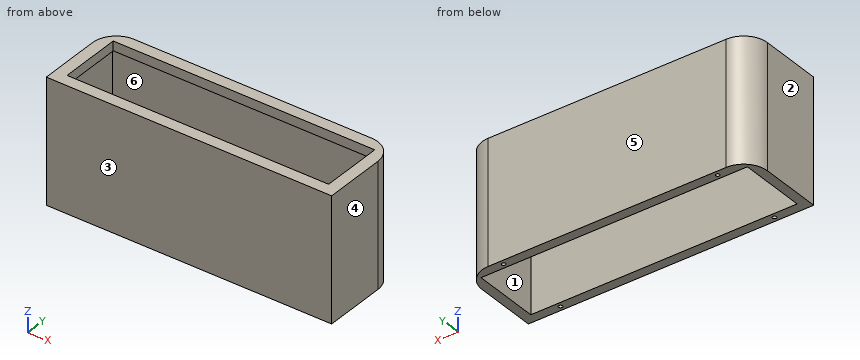
```python
from build123d import *

# Parameters (mm, degrees)
SKETCH1_W           = 152.4
SKETCH1_H           = 45.72
BOSS_EXTRUDE2_DEPTH = 66.04
SHELL1_T            = -5.08
SKETCH2_W           = 139.7
SKETCH2_H           = 33.02
CUT_EXTRUDE1_DEPTH  = 13.462
FILLET1_R           = 12.7
SKETCH4_R           = 1
CUT_EXTRUDE2_DEPTH  = 3.175


with BuildPart() as part:
    # Sketch1 → Boss-Extrude2 (new body)
    with BuildSketch(Plane.XY):
        Rectangle(SKETCH1_W, SKETCH1_H)
    extrude(amount=BOSS_EXTRUDE2_DEPTH)

    # Shell1
    shell1_openings = [part.faces().sort_by_distance(p)[0] for p in [
        (0, 0, 0),
    ]]
    offset(amount=SHELL1_T, openings=shell1_openings, kind=Kind.INTERSECTION)

    # Sketch2 → Cut-Extrude1 (cut)
    with BuildSketch(Plane.XY.offset(66.04)):
        Rectangle(SKETCH2_W, SKETCH2_H)
    extrude(amount=-CUT_EXTRUDE1_DEPTH, mode=Mode.SUBTRACT)

    # Fillet1
    fillet1_edges = [part.edges().sort_by_distance(p)[0] for p in [
        (-76.2, 22.86, 33.02),
        (76.2, 22.86, 33.02),
    ]]
    fillet(fillet1_edges, radius=FILLET1_R)

    # Sketch4 → Cut-Extrude2 (cut)
    with BuildSketch(Plane(origin=(0, 0, 0), x_dir=(-1, 0, 0), z_dir=(0, 0, -1))):
        with Locations((-57.15, -20.32)):
            Circle(SKETCH4_R)
        with Locations((-57.15, 20.32)):
            Circle(SKETCH4_R)
        with Locations((57.15, 20.32)):
            Circle(SKETCH4_R)
        with Locations((57.15, -20.32)):
            Circle(SKETCH4_R)
    extrude(amount=-CUT_EXTRUDE2_DEPTH, mode=Mode.SUBTRACT)


solid = part.part
```
Design review of the part built by this model. Coordinates are the model's own, in mm. Face numbers are marked on the shaded views. A direction names the side the tool comes from. Coordinates: 2 decimals unless noted, no trailing zeros. Loops run counter-clockwise (first coordinate to the right, second up) from the corner with the lowest first, then second, coordinate; pieces in that order, holes last. Notation, with made-up numbers: (66, 82.25) -> (85, 82.25) arc R17 cw to (85, 94.25) -> close; hole circle Ø8 at (10.5, 24.5). An arc over 180 degrees is marked (long way). Answer as a JSON object with one key per item and string values.
Q1. To check wall thickness, follow L1, parallel to Y at x = 57, z = 1; L2, parallel to X at y = -8, z = 39; L3, parallel to X at y = 20, z = 1. State the ranges of each line that lie inside material, in increasing order.
Answer block:
{"L1": "y = -22.86 to -21.31, -19.33 to -17.78, 17.78 to 19.33, 21.31 to 22.86", "L2": "x = -76.2 to -71.12, 71.12 to 76.2", "L3": "x = -71.53 to -58.1, -56.2 to 56.2, 58.1 to 71.53"}
Q2. The part is to be moulded in two halves that separate along X. For the marked faces 1, 2, 3 and 4, say which applies: +X half, -X half, draft (parallel to the pull), parting line (faces both ways), or undercut.
Answer block:
{"face 1": "undercut", "face 2": "-X half", "face 3": "draft", "face 4": "+X half"}
Q3. Take a section at C-C on y = -13. Give the boundary of the cut face in (x, z), plus the area to 3 significant figures.
Answer block:
{"outline": "(-76.2, 0) -> (-71.12, 0) -> (-71.12, 60.96) -> (-69.85, 60.96) -> (-69.85, 66.04) -> (-76.2, 66.04) -> close; (69.85, 60.96) -> (71.12, 60.96) -> (71.12, 0) -> (76.2, 0) -> (76.2, 66.04) -> (69.85, 66.04) -> close", "area": "684 mm^2"}
Q4. Take a section at A-A on z = 55. Give the boundary of the cut face in (x, y), plus the area to 3 significant figures.
Answer block:
{"outline": "(-76.2, -22.86) -> (76.2, -22.86) -> (76.2, 10.16) arc R12.7 ccw to (63.5, 22.86) -> (-63.5, 22.86) arc R12.7 ccw to (-76.2, 10.16) -> close; hole (-71.12, -17.78) -> (71.12, -17.78) -> (71.12, 17.78) -> (-71.12, 17.78) -> close", "area": "1,840 mm^2"}
Q5. Take a section at B-B on x = -20. Give the boundary of the cut face in (y, z), plus the area to 3 significant figures.
Answer block:
{"outline": "(-22.86, 0) -> (-17.78, 0) -> (-17.78, 60.96) -> (-16.51, 60.96) -> (-16.51, 66.04) -> (-22.86, 66.04) -> close; (16.51, 60.96) -> (17.78, 60.96) -> (17.78, 0) -> (22.86, 0) -> (22.86, 66.04) -> (16.51, 66.04) -> close", "area": "684 mm^2"}
Q6. Clearance check with a flat-ended pin moving along its axis: pin 1 Ø1.2 at (x, y) = (-57.15, 20.32) entering from -Z (3 decimals). State where the tip first meets the part, or that it passes through.
Answer block:
{"pin 1": "stops at z = 3.175"}
Q7. Tool access review of the marked faces 5 and 6: name each direction out of +Z, -Z, +X, -X, +Y, -Y from which nothing blocks a thin tool from reaching the whole face with its end or side.
Answer block:
{"face 5": "+Z, -Z, +X, -X, +Y", "face 6": "-Z"}
